Check sheet for the modelled part. Datum: model origin and axes. Units: mm. A direction names the side the tool comes from. Round coordinates to 2 decimals unless told otherwise and drop trailing zeros. Write each loop counter-clockwise with the first axis right and the second up, starting at its lowest first coordinate (ties: lowest second). Pieces come first, ordered by that corner, then holes. Notation, with made-up numbers: M -7.75,20 L 42.25,20 A18 cw 42.25,44 Z; hole C 89.5,29.25 d5. An arc over 180 degrees is marked long. Answer in a Markdown table with one row per item.
```python
from build123d import *

# Parameters (mm, degrees)
SKETCH1_W           = 50
SKETCH1_H           = 46.5
SKETCH1_R           = 1.75
BOSS_EXTRUDE1_DEPTH = 5
SKETCH2_R           = 11.05
CUT_EXTRUDE1_DEPTH  = 5
SKETCH3_W           = 50
SKETCH3_H           = 4
BOSS_EXTRUDE2_DEPTH = 40
RIB1_REACH          = 73.939
SKETCH4_WALL_W      = 188.304827768
SKETCH4_WALL_H      = 3
SKETCH5_W           = 5
SKETCH5_H           = 50
BOSS_EXTRUDE3_DEPTH = 27
SKETCH8_W           = 5
SKETCH8_H           = 27
BOSS_EXTRUDE5_DEPTH = 20
SKETCH9_W           = 5
SKETCH9_H           = 90
BOSS_EXTRUDE6_DEPTH = 3
BOSS_EXTRUDE7_DEPTH = 90
SKETCH12_R          = 3.5
CUT_EXTRUDE2_DEPTH  = 85.44080767
CHAMFER1_SIZE       = 7
CHAMFER2_SIZE       = 7


with BuildPart() as part:
    # Sketch1 → Boss-Extrude1 (new body)
    with BuildSketch(Plane(origin=(0, 0, 0), x_dir=(0, 0, -1), z_dir=(1, 0, 0))):
        with Locations((0, -2.25)):
            Rectangle(SKETCH1_W, SKETCH1_H)
        with Locations((15.5, 15.5)):
            Circle(SKETCH1_R, mode=Mode.SUBTRACT)
        with Locations(Location((15.5, -15.5, 0), (0, 0, 180))):
            Circle(SKETCH1_R, mode=Mode.SUBTRACT)
        with Locations((-15.5, -15.5)):
            Circle(SKETCH1_R, mode=Mode.SUBTRACT)
        with Locations(Location((-15.5, 15.5, 0), (0, 0, 180))):
            Circle(SKETCH1_R, mode=Mode.SUBTRACT)
    extrude(amount=BOSS_EXTRUDE1_DEPTH)

    # Sketch2 → Cut-Extrude1 (cut)
    with BuildSketch(Plane(origin=(5, 0, 0), x_dir=(0, 0, -1), z_dir=(1, 0, 0))):
        Circle(SKETCH2_R)
    extrude(amount=-CUT_EXTRUDE1_DEPTH, mode=Mode.SUBTRACT)

    # Sketch3 → Boss-Extrude2 (add)
    with BuildSketch(Plane(origin=(5, 0, 0), x_dir=(0, 0, -1), z_dir=(1, 0, 0))):
        with Locations((0, -23.5)):
            Rectangle(SKETCH3_W, SKETCH3_H)
    extrude(amount=BOSS_EXTRUDE2_DEPTH)

    # Sketch4 wall → Rib1 (add, up to next)
    with BuildSketch(Plane(origin=(20, -6.5, -25), x_dir=(-0.707106781187, 0.707106781187, 0), z_dir=(0.707106781187, 0.707106781187, 0)), mode=Mode.PRIVATE) as rib1_sk1:
        with Locations((0, 1.5)):
            Rectangle(SKETCH4_WALL_W, SKETCH4_WALL_H)
    rib1_tool1 = extrude(rib1_sk1.sketch, amount=-RIB1_REACH, mode=Mode.PRIVATE) - part.part
    rib1 = rib1_tool1.solids().sort_by_distance((20, -6.5, -25))[0]
    add(rib1)

    # Mirror1: Rib1 across plane
    add(rib1.mirror(Plane.XY))

    # Sketch5 → Boss-Extrude3 (add)
    with BuildSketch(Plane.XZ.offset(25.5)):
        with Locations((2.5, 0)):
            Rectangle(SKETCH5_W, SKETCH5_H)
    extrude(amount=BOSS_EXTRUDE3_DEPTH)

    # Sketch8 → Boss-Extrude5 (add)
    with BuildSketch(Plane.XY.offset(25)):
        with Locations((2.5, -39)):
            Rectangle(SKETCH8_W, SKETCH8_H)
    boss_extrude5 = extrude(amount=BOSS_EXTRUDE5_DEPTH)

    # Mirror2: Boss-Extrude5 across plane
    add(boss_extrude5.mirror(Plane.XY))

    # Sketch9 → Boss-Extrude6 (add)
    with BuildSketch(Plane.XZ.offset(52.5)):
        with Locations((2.5, 0)):
            Rectangle(SKETCH9_W, SKETCH9_H)
    extrude(amount=BOSS_EXTRUDE6_DEPTH)

    # Sketch10 → Boss-Extrude7 (add)
    with BuildSketch(Plane(origin=(0, 0, -45), x_dir=(-1, 0, 0), z_dir=(0, 0, -1))):
        with BuildLine():
            Line((25.009423753, -46.5), (25.009423753, -45.502387304))
            Line((25.009423753, -45.502387304), (13.489148599, -42.583974938))
            Line((13.489148599, -42.583974938), (0, -38.131335857))
            Line((0, -38.131335857), (0, -45.5))
            Line((0, -45.5), (0, -55.5))
            Line((0, -55.5), (25.009423753, -55.5))
            Line((25.009423753, -55.5), (25.009423753, -52.5))
            Line((25.009423753, -52.5), (15.009423753, -51.5))
            Line((15.009423753, -51.5), (9.31662479, -51.5))
            ThreePointArc((9.31662479, -51.5), (8.450599387, -51.627718677), (7.658312395, -52))
            ThreePointArc((7.658312395, -52), (3, -49.5), (7.658312395, -47))
            ThreePointArc((7.658312395, -47), (8.450599387, -47.372281323), (9.31662479, -47.5))
            Line((9.31662479, -47.5), (15.009423753, -47.5))
            Line((15.009423753, -47.5), (25.009423753, -46.5))
        make_face()
    extrude(amount=-BOSS_EXTRUDE7_DEPTH)

    # Sketch12 → Cut-Extrude2 (cut, through all)
    with BuildSketch(Plane.ZY):
        with Locations((-32, -33.5)):
            Circle(SKETCH12_R)
    cut_extrude2 = extrude(amount=-CUT_EXTRUDE2_DEPTH, mode=Mode.SUBTRACT)

    # Mirror3: Cut-Extrude2 across plane
    add(cut_extrude2.mirror(Plane.XY), mode=Mode.SUBTRACT)

    # Chamfer1
    chamfer1_edges = [part.edges().sort_by_distance(p)[0] for p in [
        (2.5, 21, -25),
    ]]
    chamfer(chamfer1_edges, length=CHAMFER1_SIZE)

    # Chamfer2
    chamfer2_edges = [part.edges().sort_by_distance(p)[0] for p in [
        (2.5, -25.5, 45),
        (2.5, -25.5, -45),
        (2.5, 21, 25),
    ]]
    chamfer(chamfer2_edges, length=CHAMFER2_SIZE)


solid = part.part
```
1. Draft check along Z on faces 1 (the face through (-20, -52, -1)), 2 (the face through (-6, -46, -45)), 3 (the face through (2.465, 13.765, 15.272)), 4 (the face through (14, -12, 22)). Enter one of: +Z half, -Z half, draft (parallel to the pull), parting line (faces both ways), or undercut.
Found:
| item | result |
|---|---|
| face 1 | draft |
| face 2 | -Z half |
| face 3 | undercut |
| face 4 | undercut |
2. Section check C-C, the plane x = 2.5. Record the cut outline in (y, z).
Found:
| item | result |
|---|---|
| outline | M -55.5,-45 L -32.5,-45 L -25.5,-38 L -25.5,-25 L 14,-25 L 21,-18 L 21,18 L 14,25 L -25.5,25 L -25.5,38 L -32.5,45 L -55.5,45 Z; hole C -33.5,-32 d7; hole C -33.5,32 d7; hole C -15.5,-15.5 d3.5; hole C -15.5,15.5 d3.5; hole C 0,0 d22.1; hole C 15.5,-15.5 d3.5; hole C 15.5,15.5 d3.5 |
3. Scan lines: L1, parallel to Y at x = 3.5, z = -15.5; L2, parallel to Z at x = 3, y = -33; L3, parallel to Y at x = 2.2, z = 32. Record each from-to range of solid material in increasing order.
Found:
| item | result |
|---|---|
| L1 | y = -55.5 to -17.25, -13.75 to 13.75, 17.25 to 21 |
| L2 | z = -45 to -35.46, -28.54 to 28.54, 35.46 to 45 |
| L3 | y = -55.5 to -37, -30 to -25.5 |
4. Section check A-A, the plane y = 0. Record the cut outline in (x, z).
Found:
| item | result |
|---|---|
| outline | M 0,-25 L 13.5,-25 L 13.5,-22 L 5,-22 L 5,-11.05 L 0,-11.05 Z; M 0,11.05 L 5,11.05 L 5,22 L 13.5,22 L 13.5,25 L 0,25 Z |
5. Section check B-B, the plane z = -15.5. Record the cut outline in (x, y), and give its area (3 significant figures).
Found:
| item | result |
|---|---|
| outline | M -25.01,-55.5 L 5,-55.5 L 5,-25.5 L 45,-25.5 L 45,-21.5 L 5,-21.5 L 5,-17.25 L 0,-17.25 L 0,-38.13 L -13.49,-42.58 L -25.01,-45.5 L -25.01,-46.5 L -15.01,-47.5 L -9.32,-47.5 A3 ccw -7.66,-47 A3 cw long -7.66,-52 A3 ccw -9.32,-51.5 L -15.01,-51.5 L -25.01,-52.5 Z; M 0,-13.75 L 5,-13.75 L 5,13.75 L 0,13.75 Z; M 0,17.25 L 5,17.25 L 5,21 L 0,21 Z |
| area | 740 mm2 |
6. Go/stop test with flat-tipped pins: pin 1 (1.5 mm diameter, centred on y = 2, z = 21.5, fed in from -X); pin 2 (5.5 mm diameter, centred on x = 3.5, z = 28.5, fed in from +Y); pin 3 (21 mm diameter, centred on y = 4, z = 9.5, fed in from +X). Record where each tip stops, or that it passes through.
Found:
| item | result |
|---|---|
| pin 1 | stops at x = 0 |
| pin 2 | stops at y = -25.5 |
| pin 3 | stops at x = 5 |
7. Section check D-D, the plane z = -32. Record the cut outline in (x, y), and give its area (3 significant figures).
Found:
| item | result |
|---|---|
| outline | M -25.01,-55.5 L 5,-55.5 L 5,-37 L 0,-37 L 0,-38.13 L -13.49,-42.58 L -25.01,-45.5 L -25.01,-46.5 L -15.01,-47.5 L -9.32,-47.5 A3 ccw -7.66,-47 A3 cw long -7.66,-52 A3 ccw -9.32,-51.5 L -15.01,-51.5 L -25.01,-52.5 Z; M 0,-30 L 5,-30 L 5,-25.5 L 0,-25.5 Z |
| area | 348 mm2 |
8. Access from +Z, -Z, +X, -X, +Y, -Y to the whole of each face (thin tool, end or side, straight path). Record for faces 5 (the face through (0, -15, -1)), 6 (the face through (2, -25.5, -31)), 7 (the face through (25, -25.5, 0)), 8 (the face through (-12, -47.5, -1)).
Found:
| item | result |
|---|---|
| face 5 | +Z, -Z, -X, +Y |
| face 6 | -Z, +X, -X, +Y |
| face 7 | +Z, -Z, +X, -Y |
| face 8 | +Z, -Z, -X |
